Work out the finished part from the listing and answer in its coordinate system (mm). A direction names the side the tool comes from. Give positions to 0.01 mm unless a question says otherwise; leave off trailing zeros.
1) Determine the mould class of faces 1 (the face through (10.382, 7.87, -19.961)), 2 (the face through (-4, 0, -4)), 3 (the face through (14, 4.8, 0)) for opening direction X: pulls with the +X half, pulls with the -X half, needs draft (parallel to the pull), parting line crosses it, or undercut.
2) Given pin 1 Ø5 at (x, y) = (7, 3.5) entering from -Z; pin 2 Ø1.1 at (y, z) = (2.5, -13.5) entering from -X; pin 3 Ø4.5 at (y, z) = (3, 1) entering from +X, each flat-ended and moving along its own axis, determine where each tip first touches the part or whether it passes through.
3) Straight lines are drawn through the part: probe 1 along X at (y, z) = (1.5, 0.5); probe 2 along Z at (x, y) = (-6.5, 1); probe 3 along X at (y, z) = (9.75, -7). For each, find the intervals that lie inside material, in ascending order.
4) A tool of negligible diameter and unlimited length cuts with its end or side. For faces 4 (the face through (5.223, 6.162, 3.704)), 5 (the face through (0, 2, 13.05)), from which of +Z, -Z, +X, -X, +Y, -Y can it reach the whole face along a straight path? Write none if from no direction.
5) Find section A-A (z = 0). Count the separate pieces of the cut face and the enclosed holes in it, plus the area to 3 significant figures.
Autodesk Inventor part; units mm, degrees
ref_plane "YZ Plane" through (0, 0, 0) normal (1, 0, 0) x (0, 1, 0)
ref_plane "XZ Plane" through (0, 0, 0) normal (0, 1, 0) x (-1, 0, 0)
ref_plane "XY Plane" through (0, 0, 0) normal (0, 0, 1) x (1, 0, 0)
sketch "Эскиз1" plane through (0, 0, 0) normal (0, 1, 0) x (-1, 0, 0)
  circle A0 centre (0, 0) radius 17.5
  dimension "d0" = 35
extrude "Выдавливание1" add sketch "Эскиз1" along normal blind 7.5
sketch "Эскиз2" plane through (0, 7.5, 0) normal (0, 1, 0) x (1, 0, 0)
  circle A0 centre (0, 0) radius 22.5
  dimension "d3" = 45
extrude "Выдавливание2" add sketch "Эскиз2" along normal blind 5
fillet "Сопряжение1" radius 4.25 1 edges at (17.5, 7.5, 0)
fillet "Сопряжение2" radius 4.25 1 edges at (-22.5, 12.5, 0)
sketch "Эскиз3" plane through (0, 0, 0) normal (0, -1, 0) x (1, 0, 0)
  line L0 (-24.85, 5.95) -> (-15.15, 5.95)
  line L1 (-15.15, 5.95) -> (-15.15, -5.95)
  line L2 (-15.15, -5.95) -> (-24.85, -5.95)
  line L3 (-24.85, -5.95) -> (-24.85, 5.95)
  line L4 (-4.7, 15.3) -> (-4.7, 25)
  line L5 (-4.7, 25) -> (5, 25)
  line L6 (5, 25) -> (5, 15.3)
  line L7 (5, 15.3) -> (-4.7, 15.3)
  line L8 (5, -15.3) -> (5, -25)
  line L9 (5, -25) -> (-4.7, -25)
  line L10 (-4.7, -25) -> (-4.7, -15.3)
  line L11 (-4.7, -15.3) -> (5, -15.3)
  line L12 (15.15, 5.95) -> (24.85, 5.95)
  line L13 (24.85, 5.95) -> (24.85, -5.95)
  line L14 (24.85, -5.95) -> (15.15, -5.95)
  line L15 (15.15, -5.95) -> (15.15, 5.95)
  circle A0 centre (0, 8) radius 2
  circle A1 centre (-5.6569, -5.6569) radius 2
  circle A2 centre (0, -8) radius 2
  circle A3 centre (0, 0) radius 4
  circle A4 centre (8, 0) radius 2
  circle A5 centre (-8, 0) radius 2
  circle A6 centre (5.6569, -5.6569) radius 2
  circle A7 centre (-5.6569, 5.6569) radius 2
  circle A8 centre (5.6569, 5.6569) radius 2
  circle A9 centre (0, 0) radius 35
extrude "Выдавливание3" cut sketch "Эскиз3" against normal through all contours A0 | A1 | A2 | A3 | A4 | A5 | A6 | A7 | A8
sketch "Эскиз4" plane through (0, 0, 0) normal (0, -1, 0) x (1, 0, 0)
  circle A0 centre (-8, 0) radius 2
  line L0 (-8, 0) -> (-13.2, 0)
  line L1 (-13.2, 0) -> (-13.2, -2)
  line L2 (-13.2, -2) -> (-15.2, -2)
  line L3 (-15.2, -2) -> (-15.2, 2)
  line L4 (-15.2, 2) -> (-13.2, 2)
  line L5 (-13.2, 2) -> (-13.2, 0)
  line L6 (2, -15.2) -> (-2, -15.2)
  line L7 (2, -13.2) -> (2, -15.2)
  line L8 (-2, -13.2) -> (0, -13.2)
  line L9 (0, -13.2) -> (2, -13.2)
  line L10 (-2, -15.2) -> (-2, -13.2)
  line L11 (15.2, 2) -> (15.2, -2)
  line L12 (13.2, 2) -> (15.2, 2)
  line L13 (13.2, -2) -> (13.2, 0)
  line L14 (13.2, 0) -> (13.2, 2)
  line L15 (15.2, -2) -> (13.2, -2)
  line L16 (-2, 15.2) -> (2, 15.2)
  line L17 (-2, 13.2) -> (-2, 15.2)
  line L18 (2, 13.2) -> (0, 13.2)
  line L19 (0, 13.2) -> (-2, 13.2)
  line L20 (2, 15.2) -> (2, 13.2)
  point P0 (0, 0)
  dimension "d10" = 5.2
  dimension "d11" = 2
  dimension "d12" = 4
  dimension "d15" = 360
extrude "Выдавливание4" add sketch "Эскиз4" along normal blind 4.5 contours L1 L2 L3 L4 L5 | L6 L10 L8 L9 L7 | L11 L15 L13 L14 L12 | L16 L20 L18 L19 L17
sketch "Эскиз6" plane through (0, 0, 0) normal (0, -1, 0) x (1, 0, 0)
  circle A0 centre (0, 0) radius 17.5
  point P0 (0, 17.5)
ref_plane "РабПлоскость1" through (0, 0, 17.5) normal (0, 0, 1) x (1, 0, 0)
sketch "Эскиз8" plane through (0, -4.5, 0) normal (0, -1, 0) x (1, 0, 0)
  line L0 (13.2, 2) -> (13.2, -2)
  line L1 (13.2, -2) -> (15.2, -2)
  line L2 (15.2, -2) -> (15.2, 2)
  line L3 (15.2, 2) -> (13.2, 2)
  line L4 (13.05, -2.15) -> (15.35, -2.15)
  line L5 (15.35, -2.15) -> (15.35, 2.15)
  line L6 (15.35, 2.15) -> (13.05, 2.15)
  line L7 (13.05, 2.15) -> (13.05, -2.15)
  line L8 (13.05, -2.15) -> (15.35, 2.15) construction
  line L9 (15.35, -2.15) -> (13.05, 2.15) construction
  line L10 (-2.15, 15.35) -> (-2.15, 13.05)
  line L11 (2.15, 15.35) -> (-2.15, 15.35)
  line L12 (2.15, 13.05) -> (2.15, 15.35)
  line L13 (-2.15, 13.05) -> (2.15, 13.05)
  line L14 (-15.35, -2.15) -> (-13.05, -2.15)
  line L15 (-15.35, 2.15) -> (-15.35, -2.15)
  line L16 (-13.05, 2.15) -> (-15.35, 2.15)
  line L17 (-13.05, -2.15) -> (-13.05, 2.15)
  line L18 (2.15, -15.35) -> (2.15, -13.05)
  line L19 (-2.15, -15.35) -> (2.15, -15.35)
  line L20 (-2.15, -13.05) -> (-2.15, -15.35)
  line L21 (2.15, -13.05) -> (-2.15, -13.05)
  point P0 (0, 0)
  point P1 (14.2, 0)
  dimension "d24" = 2.3
  dimension "d25" = 4.3
  dimension "d28" = 360
extrude "Выдавливание6" cut sketch "Эскиз8" against normal blind 9.3 contours L3 L2 L1 L0 | L7 L6 L5 L4 | L11 L12 L13 L10 | L15 L16 L17 L14 | L19 L20 L21 L18
properties part number "мини катушка 2"
Results:
1. face 1: parting line crosses it
1. face 2: needs draft
1. face 3: undercut
2. pin 1: stops at z = -17.33
2. pin 2: stops at x = -11.77
2. pin 3: stops at x = 17.98
3. probe 1: x = -17.49 to -15.35, -13.05 to -9.94, -6.06 to -3.97, 3.97 to 6.06, 9.94 to 13.05, 15.35 to 17.49
3. probe 2: z = -16.25 to -7.47, -3.84 to -1.32, 1.32 to 3.84, 7.47 to 16.25
3. probe 3: x = -21.1 to -7.14, -4.17 to -1.73, 1.73 to 4.17, 7.14 to 21.1
4. face 4: +Y, -Y
4. face 5: -Y
5. separate pieces: 4
5. enclosed holes: 0
5. area: 265 mm2
